Source: CAD feature listing. Evaluate the final solid. Frame: model axes, mm. A direction names the side the tool comes from. Round coordinates to 2 decimals unless told otherwise and drop trailing zeros. Loops run counter-clockwise (first coordinate to the right, second up) from the corner with the lowest first, then second, coordinate; pieces in that order, holes last. Notation, with made-up numbers: (46.25, -21.75) -> (54.25, -21.75) arc R23 ccw to (54.25, 6.25) -> close; hole circle Ø7 at (61.5, 82.5). An arc over 180 degrees is marked (long way). Write item = value, one per line.
from build123d import *

# Parameters (mm, degrees)
F0_W     = 32.356042
F0_H     = 1.5
F1_DEPTH = 15
F2_DEPTH = 50
F3_R     = 15
F5_DEPTH = 1.5


with BuildPart() as f1:
    # F0 (on Front) → F1 (new body)
    with BuildSketch(Plane.XZ):
        with Locations((-16.178021, 0.75)):
            Rectangle(F0_W, F0_H)
        Polygon((-32.356042, 1.5), (0, 1.5), (-4.540527, 12.738198), align=None)
    extrude(amount=F1_DEPTH)

    # F0 (on Front) → F2 (join)
    with BuildSketch(Plane.XZ):
        with Locations((-16.178021, 0.75)):
            Rectangle(F0_W, F0_H)
    extrude(amount=-F2_DEPTH)

    # F3
    f3_edges = [f1.edges().sort_by_distance(p)[0] for p in [
        (0, 50, 0.75),
        (-32.356042, 50, 0.75),
    ]]
    fillet(f3_edges, radius=F3_R)

    # F4 (on face) → F5 (cut, through all)
    with BuildSketch(Plane.XY.offset(1.5)):
        with BuildLine():
            ThreePointArc((-13.928021, 42.75), (-16.178021, 45), (-18.428021, 42.75))
            Line((-18.428021, 42.75), (-18.428021, 7.25))
            ThreePointArc((-18.428021, 7.25), (-16.178021, 5), (-13.928021, 7.25))
            Line((-13.928021, 7.25), (-13.928021, 42.75))
        make_face()
    extrude(amount=-F5_DEPTH, mode=Mode.SUBTRACT)

    # F6: F1 across face


with BuildPart() as f1_1:
    add(f1.part)
    add(f1.part.mirror(Plane(origin=(-13.1162, -15, 4.298741), x_dir=(1, 0, 0), z_dir=(0, -1, 0))))


solid = f1_1.part
1. Section query C-C (z = 11). Return the cut outline in (x, y).
Evaluation:
outline = (-8.84, -30) -> (-3.84, -30) -> (-3.84, 0) -> (-8.84, 0) -> close
2. Set-up query: faces 1 (the face through (-13, 0, 5)), 2 (the face through (-28.08, 45.49, 0.76)), 3 (the face through (-16.2, 5, 0.8)), 4 (the face through (-13, -30, 5)). Return all of +Z, -Z, +X, -X, +Y, -Y with unobstructed straight access to the full face (end or side cutting, diameter ignored); none if empty.
Evaluation:
face_1 = +Z, +X, -X, +Y
face_2 = +Z, -Z, -X, +Y
face_3 = +Z, -Z
face_4 = +Z, +X, -X, -Y
3. Line query: probe 1 along X at (y, z) = (19.5, 1); probe 2 along Z at (x, y) = (-24, -52); probe 3 along Y at (x, z) = (-3.5, 6.25). Output: solid intervals per line, ascending. Write a range as from..to.
Evaluation:
probe_1 = -32.36..-18.43, -13.93..0
probe_2 = 0..1.5
probe_3 = -30..0
4. Mould query, pull axis X, two halves, no side actions, for faces 5 (the face through (-16.1, -75, 0.8)), 6 (the face through (-18.25, -15.21, 7.2)), 7 (the face through (-4.28, 45.49, 0.76)). Classes: released by +X, released by -X, zero draft, split by the parting line, or undercut.
Evaluation:
face_5 = undercut
face_6 = released by -X
face_7 = released by +X
5. Section query B-B (x = -20.5). Return the cut outline in (y, z).
Evaluation:
outline = (-79.67, 0) -> (49.67, 0) -> (49.67, 1.5) -> (0, 1.5) -> (0, 6.29) -> (-30, 6.29) -> (-30, 1.5) -> (-79.67, 1.5) -> close
6. Contact query for flat-ended pins moving along their axis: pin 1 Ø3.5 at (x, z) = (-24, 6.5) entering from -Y; pin 2 Ø9.5 at (x, y) = (-21.5, -67.5) entering from +Z; pin 3 Ø5.5 at (x, z) = (-16.5, 6) entering from +Y. Output: stop coordinate, or through.
Evaluation:
pin_1 = -30
pin_2 = 1.5
pin_3 = 0
7. Section query A-A (y = -52). Return the cut outline in (x, z), then the cut area to 3 significant figures.
Evaluation:
outline = (-32.36, 0) -> (-18.43, 0) -> (-18.43, 1.5) -> (-32.36, 1.5) -> close; (-13.93, 0) -> (0, 0) -> (0, 1.5) -> (-13.93, 1.5) -> close
area = 41.8 mm²
8. Section query D-D (z = 4). Return the cut outline in (x, y).
Evaluation:
outline = (-26.17, -30) -> (-1.01, -30) -> (-1.01, 0) -> (-26.17, 0) -> close
